The drawing under review shows one solid part. Ordinate dimensions are in mm from its lowest x, y, z. A direction names the side the tool comes from. Round coordinates to 2 decimals unless told otherwise and drop trailing zeros. Write each loop counter-clockwise with the first axis right and the second up, starting at its lowest first coordinate (ties: lowest second). Pieces come first, ordered by that corner, then holes.
Item 1: Add section D-D (y = 115.5). Give the boundary of the cut face in (x, z).
Item 2: Add section C-C (x = 75). Give the boundary of the cut face in (y, z).
Item 3: Add section A-A (y = 510). Give the boundary of the cut face in (x, z).
Item 4: To check wall thickness, follow L1, parallel to X at y = 426, z = 43.5; L2, parallel to Y at x = 132, z = 33; L3, parallel to Y at x = 53.5, z = 19. State the ranges of each line that lie inside material, in increasing order.
Item 5: Draft analysis for pull direction Y (two halves, no side actions). For the marked faces 5, 6 and 7, state which applies: +Y half, -Y half, draft (parallel to the pull), parting line (faces both ways), or undercut.
Item 6: Clearance check with flat-ended pins moving along their axes: pin 1 Ø3 at (x, y) = (71, 229) entering from -Z; pin 2 Ø1 at (y, z) = (223.5, 41) entering from -X; pin 3 Ø1 at (y, z) = (242.5, 49) entering from -X. State where each tip first meets the part, or that it passes through.
Item 7: Add section B-B (z = 50). Give the boundary of the cut face in (x, y).
Item 8: Machinability: for the marked faces 1, 2, 3 and 4, which of the approach directions +Z, -Z, +X, -X, +Y, -Y give a long, thin tool a straight path to every point of the face, cutting with its end or side? Answer none if there is none.
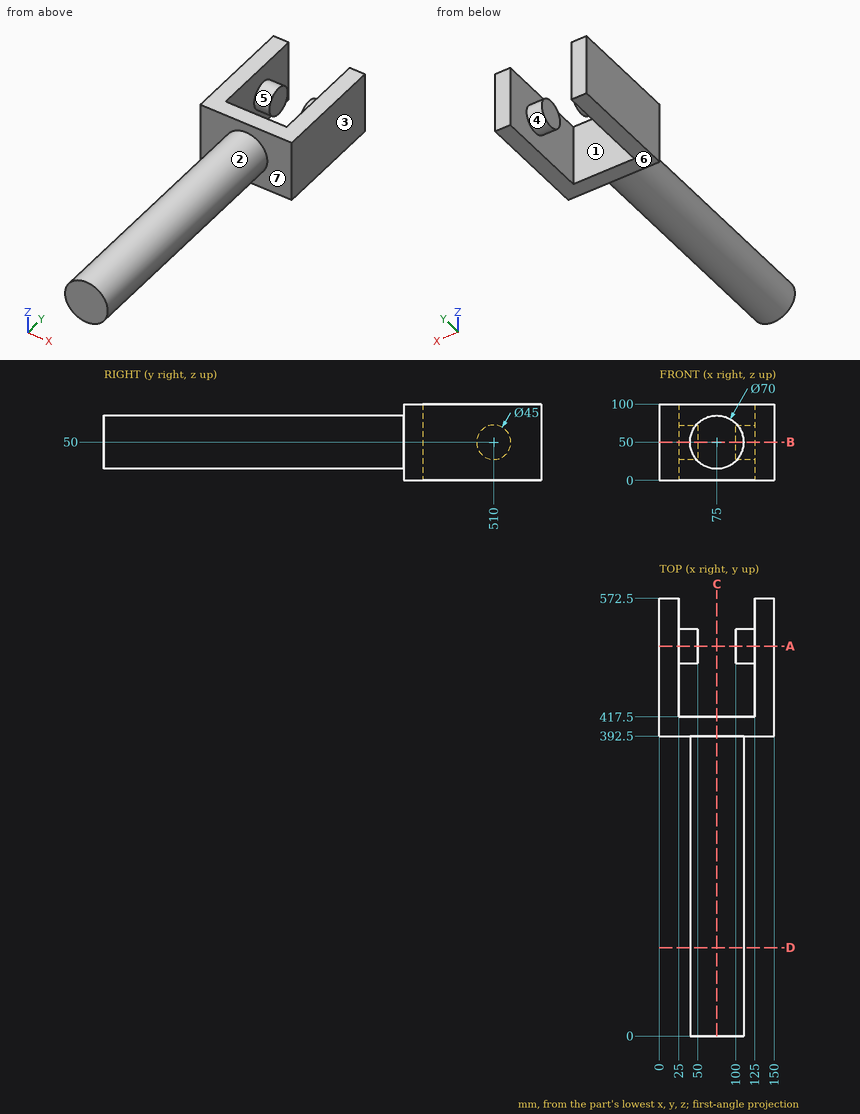
Numbers:
1. outline: circle Ø70 at (75, 50)
2. outline: (0, 15) - (392.5, 15) - (392.5, 0) - (417.5, 0) - (417.5, 100) - (392.5, 100) - (392.5, 85) - (0, 85) - close
3. outline: (0, 0) - (25, 0) - (25, 27.5) - (50, 27.5) - (50, 72.5) - (25, 72.5) - (25, 100) - (0, 100) - close; (100, 27.5) - (125, 27.5) - (125, 0) - (150, 0) - (150, 100) - (125, 100) - (125, 72.5) - (100, 72.5) - close
4. L1: x = 0 to 25, 125 to 150
4. L2: y = 392.5 to 572.5
4. L3: y = 392.5 to 417.5
5. face 5: undercut
5. face 6: draft
5. face 7: -Y half
6. pin 1: stops at z = 15.09
6. pin 2: stops at x = 41.05
6. pin 3: stops at x = 40
7. outline: (0, 392.5) - (40, 392.5) - (40, 0) - (110, 0) - (110, 392.5) - (150, 392.5) - (150, 572.5) - (125, 572.5) - (125, 532.5) - (100, 532.5) - (100, 487.5) - (125, 487.5) - (125, 417.5) - (25, 417.5) - (25, 487.5) - (50, 487.5) - (50, 532.5) - (25, 532.5) - (25, 572.5) - (0, 572.5) - close
8. face 1: +Z, -Z
8. face 2: -Y
8. face 3: +Z, -Z, +X, +Y, -Y
8. face 4: none
